Answer from the drawing. Dimensions are ordinates in mm from the lowest x, y and z of the part. Round coordinates to 2 decimals unless told otherwise and drop trailing zeros. Order: outer loops, then holes, each group sorted by start corner. A loop starts at its lowest first (then second) coordinate and runs counter-clockwise, first axis right, second up. Notation, with made-up numbers: (-9, -23) -> (49, -23) arc R13 ccw to (49, -9) -> close; hole circle Ø8 at (-2.5, 75.25). An arc over 180 degrees is marked (long way). Use a Markdown table: item, result. Add a question column.
1. Given pin 1 (5 mm diameter, centred on x = 274.5, z = 11.5, fed in from -Y), flat-ended and moving along its own axis, determine where the tip first touches the part or whether it passes through.
2. Consider L1, parallel to X at y = 347.5, z = 16.5; L2, parallel to Y at x = 277.5, z = 16.25. Determine where each line is inside the solid, lowest interval first. Write a range as [from, to].
3. Section C-C, the plane z = 11.25 is taken. Give the vertices of the cut face in (x, y), then the cut area to 3 significant figures.
4. Section B-B, the plane x = 68.5 is taken. Give the vertices of the cut face in (y, z).
5. Section A-A, the plane y = 43 is taken. Give the vertices of the cut face in (x, z).
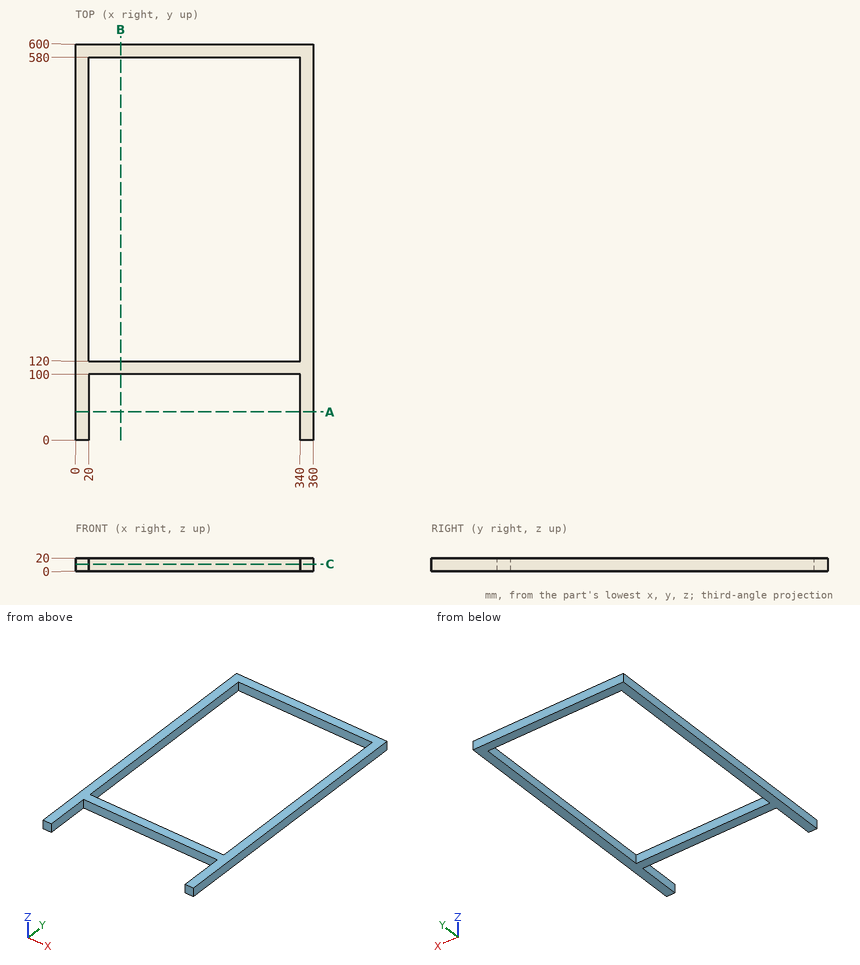
Verdict:
| question | item | result |
|---|---|---|
| 1 | pin 1 | stops at y = 100 |
| 2 | L1 | x = [0, 20], [340, 360] |
| 2 | L2 | y = [100, 120], [580, 600] |
| 3 | outline | (0, 0) -> (20, 0) -> (20, 100) -> (340, 100) -> (340, 0) -> (360, 0) -> (360, 600) -> (0, 600) -> close; hole (20, 120) -> (340, 120) -> (340, 580) -> (20, 580) -> close |
| 3 | area | 36,800 mm2 |
| 4 | outline | (100, 0) -> (120, 0) -> (120, 20) -> (100, 20) -> close; (580, 0) -> (600, 0) -> (600, 20) -> (580, 20) -> close |
| 5 | outline | (0, 0) -> (20, 0) -> (20, 20) -> (0, 20) -> close; (340, 0) -> (360, 0) -> (360, 20) -> (340, 20) -> close |
